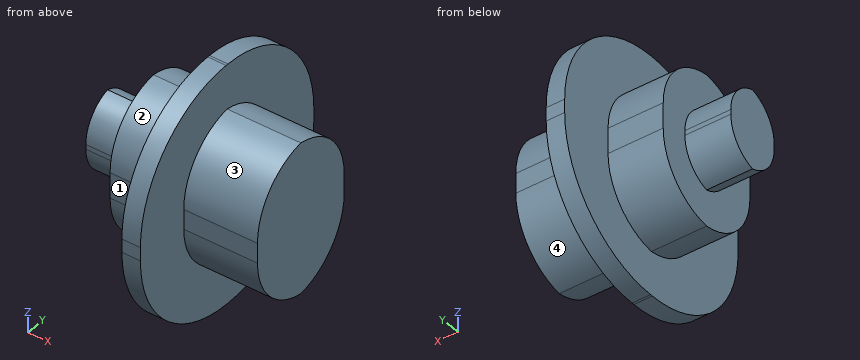
```python
from build123d import *

# Parameters (mm, degrees)
F1_DEPTH    = 25.4
F2_DEPTH    = 12.7
F3_DEPTH    = 6.35
F4_T1_DEPTH = 31.6265151256
F5_T1_DEPTH = 12.2162196785
F6_R        = 25.1416200386
F7_T1_DEPTH = 53.1085051667


# Not quite as in the source:
# - a fillet or chamfer that OpenCascade refuses, or shapes differently, is made with other operations: its cross-section is extruded or revolved along the edge and cut away or added


with BuildPart() as f1:
    # F0 (on Front) → F1 (new body, symmetric)
    with BuildSketch(Plane.XZ):
        Polygon((-20.4155612737, 26.5935901552), (-20.4155612737, 16.8710052967), (-20.4155612737, -16.9768668711), (-20.4155612737, -26.6668144614), (-16.3158904761, -26.6668144614), (-16.3158904761, -16.9768668711), (-16.3158904761, 16.8710052967), (-16.3158904761, 26.5935901552), align=None)
    extrude(amount=F1_DEPTH, both=True)

    # F0 (on Front) → F2 (join, symmetric)
    with BuildSketch(Plane.XZ):
        Polygon((-32.6317809522, 16.8710052967), (-32.6317809522, 9.0427109972), (-32.6317809522, -9.1775488108), (-32.6317809522, -16.9768668711), (-20.4155612737, -16.9768668711), (-20.4155612737, 16.8710052967), align=None)
        Polygon((0, 16.8710052967), (-16.3158904761, 16.8710052967), (-16.3158904761, -16.9768668711), (0, -16.9768668711), (0, -9.1775488108), (0, 0), (0, 9.0427109972), align=None)
    extrude(amount=F2_DEPTH, both=True)

    # F0 (on Front) → F3 (join, symmetric)
    with BuildSketch(Plane.XZ):
        Polygon((-32.6317809522, -9.1775488108), (-32.6317809522, 9.0427109972), (-42.7959375083, 9.0427109972), (-42.7959375083, 0), (-42.7959375083, -9.1775488108), align=None)
    extrude(amount=F3_DEPTH, both=True)

    # F4: fillet of radius 8.5849434278 on 4 edges, made by hand

    # F4_s2 → F4_t1 (cut)
    with BuildSketch(Plane.YZ.offset(-64.2582960778)):
        with BuildLine():
            ThreePointArc((-6.35, 0.4577675694), (-3.8355282861, 6.5282392833), (2.2349434278, 9.0427109972))
            Line((2.2349434278, 9.0427109972), (-6.35, 9.0427109972))
            Line((-6.35, 9.0427109972), (-6.35, 0.4577675694))
        make_face()
        with BuildLine():
            ThreePointArc((2.2349434278, -9.1775488108), (-3.8355282861, -6.6630770969), (-6.35, -0.592605383))
            Line((-6.35, -0.592605383), (-6.35, -9.1775488108))
            Line((-6.35, -9.1775488108), (2.2349434278, -9.1775488108))
        make_face()
        with BuildLine():
            ThreePointArc((-2.2349434278, 9.0427109972), (3.8355282861, 6.5282392833), (6.35, 0.4577675694))
            Line((6.35, 0.4577675694), (6.35, 9.0427109972))
            Line((6.35, 9.0427109972), (-2.2349434278, 9.0427109972))
        make_face()
        with BuildLine():
            ThreePointArc((-2.2349434278, -9.1775488108), (3.8355282861, -6.6630770969), (6.35, -0.592605383))
            Line((6.35, -0.592605383), (6.35, -9.1775488108))
            Line((6.35, -9.1775488108), (-2.2349434278, -9.1775488108))
        make_face()
    extrude(amount=F4_T1_DEPTH, mode=Mode.SUBTRACT)

    # F5: fillet of radius 14.1038356314 on 4 edges, made by hand

    # F5_s2 → F5_t1 (cut)
    with BuildSketch(Plane.YZ.offset(-32.6317809522)):
        with BuildLine():
            ThreePointArc((-1.4038356314, 16.8710052967), (8.5690821843, 12.740087481), (12.7, 2.7671696653))
            Line((12.7, 2.7671696653), (12.9820767126, 2.7671696653))
            Line((12.9820767126, 2.7671696653), (12.9820767126, 17.1530820093))
            Line((12.9820767126, 17.1530820093), (-1.4038356314, 17.1530820093))
            Line((-1.4038356314, 17.1530820093), (-1.4038356314, 16.8710052967))
        make_face()
        with BuildLine():
            ThreePointArc((12.7, -2.8730312397), (8.5690821843, -12.8459490554), (-1.4038356314, -16.9768668711))
            Line((-1.4038356314, -16.9768668711), (-1.4038356314, -17.2589435837))
            Line((-1.4038356314, -17.2589435837), (12.9820767126, -17.2589435837))
            Line((12.9820767126, -17.2589435837), (12.9820767126, -2.8730312397))
            Line((12.9820767126, -2.8730312397), (12.7, -2.8730312397))
        make_face()
        with BuildLine():
            ThreePointArc((1.4038356314, 16.8710052967), (-8.5690821843, 12.740087481), (-12.7, 2.7671696653))
            Line((-12.7, 2.7671696653), (-12.9820767126, 2.7671696653))
            Line((-12.9820767126, 2.7671696653), (-12.9820767126, 17.1530820093))
            Line((-12.9820767126, 17.1530820093), (1.4038356314, 17.1530820093))
            Line((1.4038356314, 17.1530820093), (1.4038356314, 16.8710052967))
        make_face()
        with BuildLine():
            ThreePointArc((1.4038356314, -16.9768668711), (-8.5690821843, -12.8459490554), (-12.7, -2.8730312397))
            Line((-12.7, -2.8730312397), (-12.9820767126, -2.8730312397))
            Line((-12.9820767126, -2.8730312397), (-12.9820767126, -17.2589435837))
            Line((-12.9820767126, -17.2589435837), (1.4038356314, -17.2589435837))
            Line((1.4038356314, -17.2589435837), (1.4038356314, -16.9768668711))
        make_face()
    extrude(amount=F5_T1_DEPTH, mode=Mode.SUBTRACT)

    # F6
    f6_edges = [f1.edges().sort_by_distance(p)[0] for p in [
        (-18.365726, -25.4, 26.59359),
        (-18.365726, -25.4, -26.666814),
        (-18.365726, 25.4, 26.59359),
        (-18.365726, 25.4, -26.666814),
    ]]
    fillet(f6_edges, radius=F6_R)

    # F7: fillet of radius 14.7170458762 on 4 edges, made by hand

    # F7_s2 → F7_t1 (cut)
    with BuildSketch(Plane.YZ.offset(-16.3158904761)):
        with BuildLine():
            ThreePointArc((-2.0170458762, 16.8710052967), (8.3894770619, 12.5604823586), (12.7, 2.1539594205))
            Line((12.7, 2.1539594205), (12.7, 16.8710052967))
            Line((12.7, 16.8710052967), (-2.0170458762, 16.8710052967))
        make_face()
        with BuildLine():
            ThreePointArc((-2.0170458762, -16.9768668711), (8.3894770619, -12.666343933), (12.7, -2.2598209949))
            Line((12.7, -2.2598209949), (12.7, -16.9768668711))
            Line((12.7, -16.9768668711), (-2.0170458762, -16.9768668711))
        make_face()
        with BuildLine():
            ThreePointArc((2.0170458762, 16.8710052967), (-8.3894770619, 12.5604823586), (-12.7, 2.1539594205))
            Line((-12.7, 2.1539594205), (-12.7, 16.8710052967))
            Line((-12.7, 16.8710052967), (2.0170458762, 16.8710052967))
        make_face()
        with BuildLine():
            ThreePointArc((-12.7, -2.2598209949), (-8.3894770619, -12.666343933), (2.0170458762, -16.9768668711))
            Line((2.0170458762, -16.9768668711), (-12.7, -16.9768668711))
            Line((-12.7, -16.9768668711), (-12.7, -2.2598209949))
        make_face()
    extrude(amount=F7_T1_DEPTH, mode=Mode.SUBTRACT)


solid = f1.part
```
The model under review builds one solid part; all positions refer to its coordinate system, in mm. Face numbers are marked on the shaded views. A direction names the side the tool comes from. Coordinates: 2 decimals unless noted, no trailing zeros. Loops run counter-clockwise (first coordinate to the right, second up) from the corner with the lowest first, then second, coordinate; pieces in that order, holes last. Notation, with made-up numbers: (-22.5, 64.5) -> (-9.5, 64.5) arc R23 ccw to (-9.5, 88.5) -> close; hole circle Ø7 at (35, 7.25). An arc over 180 degrees is marked (long way). Answer as CSV lines item,"result".
Item 1: Take a section at B-B, the plane y = 1. State the section outline as (x, z) points.
Results below:
outline,"(-42.8, -8.54) -> (-32.63, -8.54) -> (-32.63, -16.77) -> (-20.42, -16.77) -> (-20.42, -26.66) -> (-16.32, -26.66) -> (-16.32, -16.66) -> (0, -16.66) -> (0, 16.56) -> (-16.32, 16.56) -> (-16.32, 26.58) -> (-20.42, 26.58) -> (-20.42, 16.66) -> (-32.63, 16.66) -> (-32.63, 8.41) -> (-42.8, 8.41) -> close"
Item 2: Insertion check: pin 1 (4 mm diameter, centred on x = -28, y = 7.5, fed in from +Z); pin 2 (6 mm diameter, centred on x = -25.5, z = -1, fed in from +Y); pin 3 (1 mm diameter, centred on y = 14, z = -5.5, fed in from +X). Each pin has a flat end and moves straight along its axis. Give the tip position at first contact, or say it passes through.
Results below:
pin 1,"stops at z = 15.07"
pin 2,"stops at y = 12.7"
pin 3,"stops at x = -16.32"
Item 3: For L1, parallel to X at y = -21.5, z = 13; L2, parallel to X at y = 11.5, z = -7.5; L3, parallel to Z at x = -18, y = 11.5, list the stretches that pass through material, from the lowest coordinate up.
Results below:
L1,"x = -20.42 to -16.32"
L2,"x = -32.63 to 0"
L3,"z = -24.01 to 23.94"
Item 4: Machinability: for the marked faces 1, 2, 3 and 4, which of the approach directions +Z, -Z, +X, -X, +Y, -Y give a long, thin tool a straight path to every point of the face, cutting with its end or side? Answer none if there is none.
Results below:
face 1,"+Z, -Z, -X, -Y"
face 2,"+Z, -X, -Y"
face 3,"+Z, +X, -Y"
face 4,"-Z, +X, +Y"
Item 5: Take a section at D-D, the plane z = 10.5. State the section outline as (x, y) points.
Results below:
outline,"(-32.63, -10.39) -> (-20.42, -10.39) -> (-20.42, -23.72) -> (-16.32, -23.72) -> (-16.32, -10.1) -> (0, -10.1) -> (0, 10.1) -> (-16.32, 10.1) -> (-16.32, 23.72) -> (-20.42, 23.72) -> (-20.42, 10.39) -> (-32.63, 10.39) -> close"
Item 6: Take a section at A-A, the plane z = -14.5. State the section outline as (x, y) points.
Results below:
outline,"(-32.63, -6.58) -> (-20.42, -6.58) -> (-20.42, -21.79) -> (-16.32, -21.79) -> (-16.32, -6.15) -> (0, -6.15) -> (0, 6.15) -> (-16.32, 6.15) -> (-16.32, 21.79) -> (-20.42, 21.79) -> (-20.42, 6.58) -> (-32.63, 6.58) -> close"
Item 7: Take a section at C-C, the plane x = -8. State the section outline as (y, z) points.
Results below:
outline,"(-12.7, -2.26) arc R14.72 ccw to (0, -16.84) arc R14.72 ccw to (12.7, -2.26) -> (12.7, 2.15) arc R14.72 ccw to (0, 16.73) arc R14.72 ccw to (-12.7, 2.15) -> close"
